from build123d import *

# Parameters (mm, degrees)
SKETCH1_W                 = 6
SKETCH1_H                 = 6
BOSS_EXTRUDE1_DEPTH       = 49
F_2_0MM_DOWEL_HOLE1_D     = 2
F_2_0MM_DOWEL_HOLE1_DEPTH = 10
F_2_0MM_DOWEL_HOLE1_TIP   = 0.600860619
F_2_0MM_DOWEL_HOLE8_D     = 2
F_2_0MM_DOWEL_HOLE8_DEPTH = 10
F_2_0MM_DOWEL_HOLE8_TIP   = 0.600860619


with BuildPart() as part:
    # Sketch1 → Boss-Extrude1 (new body)
    with BuildSketch(Plane(origin=(0, 0, 0), x_dir=(0, 0, -1), z_dir=(1, 0, 0))):
        Rectangle(SKETCH1_W, SKETCH1_H)
    extrude(amount=BOSS_EXTRUDE1_DEPTH)

    # Ø2.0mm Dowel Hole1
    with Locations(Plane(origin=(11.5, 0, 3), x_dir=(0, 1, 0), z_dir=(0, 0, 1))):
        with Locations((0, 0), (0, -26)):
            Hole(F_2_0MM_DOWEL_HOLE1_D / 2, depth=F_2_0MM_DOWEL_HOLE1_DEPTH)
            with Locations((0, 0, -(F_2_0MM_DOWEL_HOLE1_DEPTH + F_2_0MM_DOWEL_HOLE1_TIP / 2))):  # 118° drill point
                Cone(0, F_2_0MM_DOWEL_HOLE1_D / 2, F_2_0MM_DOWEL_HOLE1_TIP, mode=Mode.SUBTRACT)

    # Ø2.0mm Dowel Hole8
    with Locations(Plane(origin=(8.5, 3, 0), x_dir=(0, 0, 1), z_dir=(0, 1, 0))):
        with Locations((0, 0), (0, 32)):
            Hole(F_2_0MM_DOWEL_HOLE8_D / 2, depth=F_2_0MM_DOWEL_HOLE8_DEPTH)
            with Locations((0, 0, -(F_2_0MM_DOWEL_HOLE8_DEPTH + F_2_0MM_DOWEL_HOLE8_TIP / 2))):  # 118° drill point
                Cone(0, F_2_0MM_DOWEL_HOLE8_D / 2, F_2_0MM_DOWEL_HOLE8_TIP, mode=Mode.SUBTRACT)


solid = part.part
Work out the finished part from the listing and answer in its coordinate system (mm). Coordinates: 2 decimals unless noted, no trailing zeros. Loops run counter-clockwise (first coordinate to the right, second up) from the corner with the lowest first, then second, coordinate; pieces in that order, holes last. Notation, with made-up numbers: (60.25, 51.5) -> (73.25, 51.5) arc R17 cw to (73.25, 84.5) -> close; hole circle Ø11 at (-16, 4.25). An arc over 180 degrees is marked (long way). Write each question's results on one line, items separated by ' | '. Start each with the question number.
1) Find section C-C on z = 0. Determine the outline of the cut face in (x, y), then the cut area to 3 significant figures.
2) A flat-ended cylindrical pin translates along its axis: P1, Ø3, axis at x = 37.5, y = 0, coming from the +Z side. Find the tip coordinate at first contact, or state that the pin passes through.
3) The mould has two halves that part along Z. Classify faces 1 (the cylindrical face through (41.49, -0.04, 0.13)), 2 (the flat face through (24, 0, -3)), 3 (the flat face through (0, 0, 0)), 4 (the cylindrical face through (9.49, -0.04, 0.13)): pulls with the +Z half, pulls with the -Z half, needs draft (parallel to the pull), parting line crosses it, or undercut.
4) Find section B-B on x = 40.5. Determine the outline of the cut face in (y, z).
5) Find section A-A on y = 0. Determine the outline of the cut face in (x, z).
6) Consider line 1 along X through (y, z) = (-1.45, 0); line 2 along X through (y, z) = (0.1, 1.6); line 3 along Y through (x, z) = (11.5, 1.45). Determine where each line is inside the solid, lowest interval first.
7) Find section D-D on z = 2.35. Determine the outline of the cut face in (x, y).
Response values:
1) outline: (0, -3) -> (7.5, -3) -> (7.5, 3) -> (0, 3) -> close; (9.5, -3) -> (39.5, -3) -> (39.5, 3) -> (9.5, 3) -> close; (41.5, -3) -> (49, -3) -> (49, 3) -> (41.5, 3) -> close; hole circle Ø2 at (11.5, 0); hole circle Ø2 at (37.5, 0) | area: 264 mm^2
2) P1: stops at z = 3
3) face 1: undercut | face 2: pulls with the -Z half | face 3: needs draft | face 4: undercut
4) outline: (-3, -3) -> (3, -3) -> (3, -1) -> (-3, -1) -> close; (-3, 1) -> (3, 1) -> (3, 3) -> (-3, 3) -> close
5) outline: (0, -3) -> (10.5, -3) -> (10.5, 3) -> (0, 3) -> close; (12.5, -3) -> (36.5, -3) -> (36.5, 3) -> (12.5, 3) -> close; (38.5, -3) -> (49, -3) -> (49, 3) -> (38.5, 3) -> close; hole circle Ø2 at (8.5, 0); hole circle Ø2 at (40.5, 0)
6) line 1: x = 0 to 7.5, 9.5 to 39.5, 41.5 to 49 | line 2: x = 0 to 10.51, 12.49 to 36.51, 38.49 to 49 | line 3: y = -3 to -1, 1 to 3
7) outline: (0, -3) -> (49, -3) -> (49, 3) -> (0, 3) -> close; hole circle Ø2 at (11.5, 0); hole circle Ø2 at (37.5, 0)
